Model file for the job. Use its own axes, mm. Face numbers are marked on the shaded views. Coordinates: 2 decimals unless noted, no trailing zeros. Loops run counter-clockwise (first coordinate to the right, second up) from the corner with the lowest first, then second, coordinate; pieces in that order, holes last. Notation, with made-up numbers: M -1.5,11.25 L 27.5,11.25 A16 ccw 27.5,15.25 Z; hole C 86,-1 d5. An arc over 180 degrees is marked long. Write item = value, one per line. Start each with the question number.
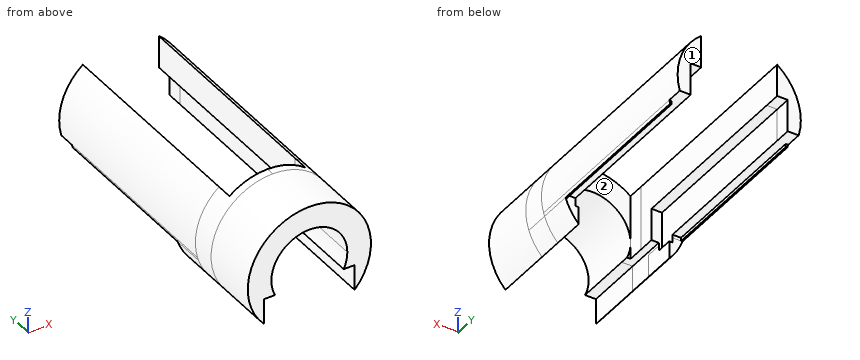
from build123d import *
from build123d.topology import SkipClean

# Parameters (mm, degrees)
SKETCH1_R            = 38.1
BOSS_EXTRUDE5_DEPTH  = 5
BOSS_EXTRUDE6_DEPTH  = 10
BOSS_EXTRUDE7_DEPTH  = 130
SKETCH6_W            = 60
SKETCH6_H            = 10
CUT_EXTRUDE1_DEPTH   = 20
SKETCH7_W            = 1.51134539
SKETCH7_H            = 120
BOSS_EXTRUDE8_DEPTH  = 2
SKETCH8_OUTSIDE_W    = 114.332
SKETCH8_OUTSIDE_H    = 114.332
SKETCH8_OUTSIDE_R    = 38.1
CUT_EXTRUDE2_DEPTH   = 155.687491414
SKETCH10_W           = 70.5
SKETCH10_H           = 2
BOSS_EXTRUDE9_DEPTH  = 20
SKETCH11_W           = 56
SKETCH11_H           = 30
CUT_EXTRUDE3_DEPTH   = 123.487632029
BOSS_EXTRUDE10_START = 35
BOSS_EXTRUDE10_DEPTH = 35
SKETCH13_R           = 23.5
CUT_EXTRUDE4_DEPTH   = 151.010732949
BOSS_EXTRUDE11_DEPTH = 20
SKETCH16_W           = 60
SKETCH16_H           = 25
CUT_EXTRUDE5_DEPTH   = 110


with BuildPart() as part:
    # Sketch1 → Boss-Extrude5 (new body)
    with BuildSketch(Plane(origin=(0, 0, 0), x_dir=(1, 0, 0), z_dir=(0, 1, 0))):
        with Locations(Location((0, 0, 0), (0, 0, 270))):
            Circle(SKETCH1_R)
    extrude(amount=BOSS_EXTRUDE5_DEPTH)

    # Sketch4 → Boss-Extrude6 (add)
    with BuildSketch(Plane(origin=(0, 5, 0), x_dir=(1, 0, 0), z_dir=(0, 1, 0))):
        with BuildLine():
            ThreePointArc((38.1, 0), (-16.677229986, 34.256094348), (-23.5, -29.989331436))
            Line((-23.5, -29.989331436), (-23.5, 10.010668564))
            Line((-23.5, 10.010668564), (23.5, 10.010668564))
            Line((23.5, 10.010668564), (23.5, -29.989331436))
            ThreePointArc((23.5, -29.989331436), (34.256094348, -16.677229986), (38.1, 0))
        make_face()
    extrude(amount=BOSS_EXTRUDE6_DEPTH)

    # Sketch5 → Boss-Extrude7 (add)
    with SkipClean():  # the faces are left unmerged after this step: merging them gives an invalid solid
        with BuildSketch(Plane(origin=(0, 15, 0), x_dir=(1, 0, 0), z_dir=(0, 1, 0))):
            with BuildLine():
                Line((-23.5, 10.010668564), (-36.76134539, 10.010668564))
                ThreePointArc((-36.76134539, 10.010668564), (-36.164311649, -11.98968569), (-23.5, -29.989331436))
                Line((-23.5, -29.989331436), (-23.5, 10.010668564))
            make_face()
            with BuildLine():
                Line((23.5, 10.010668564), (36.76134539, 10.010668564))
                ThreePointArc((36.76134539, 10.010668564), (36.164311649, -11.98968569), (23.5, -29.989331436))
                Line((23.5, -29.989331436), (23.5, 10.010668564))
            make_face()
        extrude(amount=BOSS_EXTRUDE7_DEPTH)

    # Sketch6 → Cut-Extrude1 (cut)
    with SkipClean():  # the faces are left unmerged after this step: merging them gives an invalid solid
        with BuildSketch(Plane(origin=(0, 0, -10.010668564), x_dir=(-1, 0, 0), z_dir=(0, 0, -1))):
            with Locations((0, 140)):
                Rectangle(SKETCH6_W, SKETCH6_H)
        extrude(amount=-CUT_EXTRUDE1_DEPTH, mode=Mode.SUBTRACT)

    # Sketch7 → Boss-Extrude8 (add)
    with SkipClean():  # the faces are left unmerged after this step: merging them gives an invalid solid
        with BuildSketch(Plane(origin=(0, 0, -10.010668564), x_dir=(-1, 0, 0), z_dir=(0, 0, -1))):
            with Locations((36.005672695, 75)):
                Rectangle(SKETCH7_W, SKETCH7_H)
            with Locations((-36.005672695, 75)):
                Rectangle(SKETCH7_W, SKETCH7_H)
        extrude(amount=BOSS_EXTRUDE8_DEPTH)

    # Sketch8 outside → Cut-Extrude2 (cut, through all)
    with SkipClean():  # the faces are left unmerged after this step: merging them gives an invalid solid
        with BuildSketch(Plane.XZ):
            Rectangle(SKETCH8_OUTSIDE_W, SKETCH8_OUTSIDE_H)
            with Locations(Location((0, 0, 0), (0, 0, 341.624658097))):
                Circle(SKETCH8_OUTSIDE_R, mode=Mode.SUBTRACT)
        extrude(amount=-CUT_EXTRUDE2_DEPTH, mode=Mode.SUBTRACT)
    add(part.part.scale(1), mode=Mode.REPLACE)  # the faces are merged on a copy

    # Sketch10 → Boss-Extrude9 (add)
    with SkipClean():  # the faces are left unmerged after this step: merging them gives an invalid solid
        with BuildSketch(Plane(origin=(0, 15, 0), x_dir=(1, 0, 0), z_dir=(0, 1, 0))):
            with Locations((0, 11.010668564)):
                Rectangle(SKETCH10_W, SKETCH10_H)
        extrude(amount=BOSS_EXTRUDE9_DEPTH)

    # Sketch11 → Cut-Extrude3 (cut, through all)
    with SkipClean():  # the faces are left unmerged after this step: merging them gives an invalid solid
        with BuildSketch(Plane(origin=(0, 35, 0), x_dir=(1, 0, 0), z_dir=(0, 1, 0))):
            with Locations((0, 25.010668564)):
                Rectangle(SKETCH11_W, SKETCH11_H)
        extrude(amount=-CUT_EXTRUDE3_DEPTH, mode=Mode.SUBTRACT)

    # Sketch12 → Boss-Extrude10 (add)
    with SkipClean():  # the faces are left unmerged after this step: merging them gives an invalid solid
        with BuildSketch(Plane.XZ.offset(BOSS_EXTRUDE10_START)):
            with BuildLine():
                Line((-28, -25.838150089), (-28, -10.010668564))
                Line((-28, -10.010668564), (28, -10.010668564))
                Line((28, -10.010668564), (28, -25.838150089))
                ThreePointArc((28, -25.838150089), (0, 38.1), (-28, -25.838150089))
            make_face()
        extrude(amount=-BOSS_EXTRUDE10_DEPTH)

    # Sketch13 → Cut-Extrude4 (cut, through all)
    with SkipClean():  # the faces are left unmerged after this step: merging them gives an invalid solid
        with BuildSketch(Plane(origin=(0, 5, 0), x_dir=(1, 0, 0), z_dir=(0, 1, 0))):
            Circle(SKETCH13_R)
        extrude(amount=-CUT_EXTRUDE4_DEPTH, mode=Mode.SUBTRACT)

    # Sketch14 → Boss-Extrude11 (add)
    with SkipClean():  # the faces are left unmerged after this step: merging them gives an invalid solid
        with BuildSketch(Plane(origin=(0, 15, 0), x_dir=(1, 0, 0), z_dir=(0, 1, 0))):
            with BuildLine():
                Line((28, 25.838150089), (28, 12.010668564))
                Line((28, 12.010668564), (36.157348363, 12.010668564))
                ThreePointArc((36.157348363, 12.010668564), (32.815257862, 19.35894758), (28, 25.838150089))
            make_face()
            with BuildLine():
                Line((-28, 12.010668564), (-28, 25.838150089))
                ThreePointArc((-28, 25.838150089), (-32.815257862, 19.35894758), (-36.157348363, 12.010668564))
                Line((-36.157348363, 12.010668564), (-28, 12.010668564))
            make_face()
        extrude(amount=BOSS_EXTRUDE11_DEPTH)

    # Sketch16 → Cut-Extrude5 (cut)
    with SkipClean():  # the faces are left unmerged after this step: merging them gives an invalid solid
        with BuildSketch(Plane(origin=(0, 135, 0), x_dir=(1, 0, 0), z_dir=(0, 1, 0))):
            with Locations((0, 2.510668564)):
                Rectangle(SKETCH16_W, SKETCH16_H)
        extrude(amount=-CUT_EXTRUDE5_DEPTH, mode=Mode.SUBTRACT)


solid = part.part
Item 1: Pull direction X, two halves, no side cores. Call the marked faces 1 and 2: +X half, -X half, draft (parallel to the pull), parting line (faces both ways), or undercut.
Item 2: Probe L1, parallel to X at y = -6, z = 0; L2, parallel to Y at x = -13, z = 28; L3, parallel to X at y = 63, z = 0. List the from-to ranges inside material, lowest first.
Item 3: Pin check, flat tips, straight feed: pin 1 Ø9 at (x, z) = (33.5, -19.5) entering from +Y; pin 2 Ø3.5 at (x, y) = (26, 8) entering from -Z; pin 3 Ø17.5 at (y, z) = (6.5, -15) entering from -X. Stop position of each tip, or through.
Item 4: Cut at C-C (x = -16.5). Give the cut face in (y, z).
Item 5: Cut at D-D (z = 8). Give the cut face in (x, y), plus the area to 3 significant figures.
Item 6: Cut at A-A (y = 128.5). Give the cut face in (x, z), plus the area to 3 significant figures.
Item 7: Cut at B-B (z = -3). Give the cut face in (x, y), plus the area to 3 significant figures.
Reported:
q1.face_1 = draft
q1.face_2 = undercut
q2.L1 = -38.1 to -23.5, 23.5 to 38.1
q2.L2 = -35 to 5
q2.L3 = -38.1 to -30, 30 to 38.1
q3.pin_1 = 35
q3.pin_2 = -10.01
q3.pin_3 = -37.58
q4.outline = M -35,16.73 L 5,16.73 L 5,34.34 L -35,34.34 Z
q5.outline = M -37.25,-35 L -22.1,-35 L -22.1,5 L -23.5,5 L -23.5,25 L -30,25 L -30,145 L -37.25,145 Z; M 22.1,-35 L 37.25,-35 L 37.25,145 L 30,145 L 30,25 L 23.5,25 L 23.5,5 L 22.1,5 Z
q5.area = 3,500 mm^2
q6.outline = M -36.16,-12.01 L -35.25,-12.01 L -35.25,-10.01 L -30,-10.01 L -30,9.99 L -23.5,9.99 L -23.5,29.99 A38.1 ccw Z; M 23.5,9.99 L 30,9.99 L 30,-10.01 L 35.25,-10.01 L 35.25,-12.01 L 36.16,-12.01 A38.1 ccw 23.5,29.99 Z
q6.area = 639 mm^2
q7.outline = M -37.98,-35 L -23.31,-35 L -23.31,5 L -23.5,5 L -23.5,25 L -30,25 L -30,145 L -37.98,145 Z; M 23.31,-35 L 37.98,-35 L 37.98,145 L 30,145 L 30,25 L 23.5,25 L 23.5,5 L 23.31,5 Z
q7.area = 3,670 mm^2
